Here's the drawing with two shaded views (mm, measured from the low corner). I have some questions. Give positions to 0.01 mm unless a question says otherwise; leave off trailing zeros. Write each loop counter-clockwise with the first axis right and the second up, starting at its lowest first coordinate (ties: lowest second). Pieces come first, ordered by that corner, then holes. Notation, with made-up numbers: (55.5, 54.5) - (90.5, 54.5) arc R38 cw to (90.5, 92.5) - close; hole circle Ø7 at (14, -31). An arc over 180 degrees is marked (long way). Answer as CSV lines item,"result". Start each with the question number.
Q1. Imagine slicing it at A-A on y = 17.5. List the corners of the cut face in (x, z) for me.
Q2. Will these pins go through, and if not, where does the flat tip stop? pin 1 Ø8 at (x, z) = (10, 7.5) entering from -Y; pin 2 Ø1.5 at (x, y) = (53, 35) entering from +Z (1 decimal); pin 3 Ø2 at (x, z) = (52, 21.5) entering from +Y; pin 4 Ø10 at (x, y) = (49.5, 12.5) entering from +Z (1 decimal).
Q3. Imagine slicing it at D-D on y = 7.5. List the corners of the cut face in (x, z) for me (1 decimal).
Q4. Imagine slicing it at C-C on x = 50. List the corners of the cut face in (y, z) for me.
Q5. If I drill on line 1 along Y through (x, z) = (29.5, 26); line 2 along X through (y, z) = (50.5, 18) (1 decimal); line 3 along X through (y, z) = (4, 4.5) (1 decimal), over which ranges is the centre line in solid material (lowest first)?
Q6. Imagine slicing it at B-B on z = 41. List the corners of the cut face in (x, y) for me (1 decimal).
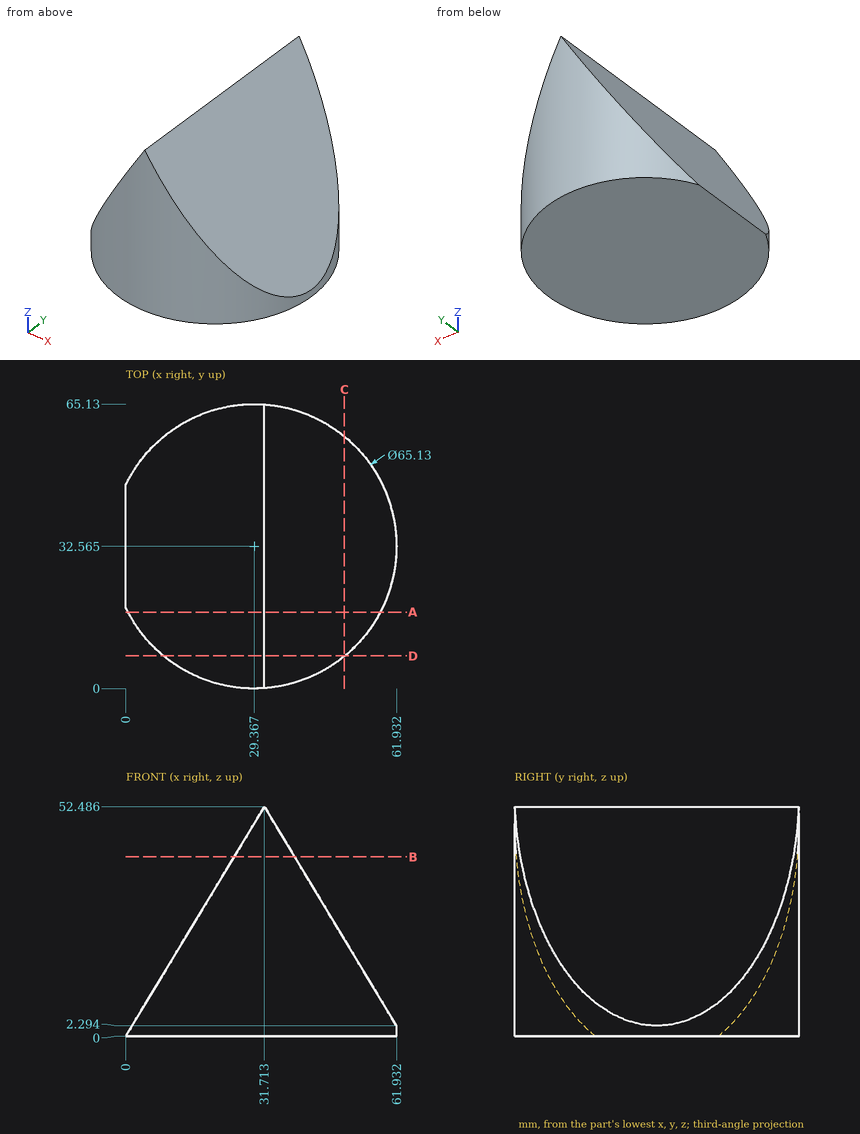
Conclusion:
1,outline,"(0.5, 0) - (58.24, 0) - (58.24, 8.43) - (31.71, 52.49) - (0.5, 0.82) - close"
2,pin 1,"y = 3.85"
2,pin 2,"z = 18.4"
2,pin 3,"through"
2,pin 4,"z = 31.2"
3,outline,"(8.6, 0) - (50.2, 0) - (50.2, 21.9) - (31.7, 52.5) - (8.6, 14.2) - close"
4,outline,"(7.37, 0) - (57.76, 0) - (57.76, 22.11) - (7.37, 22.11) - close"
5,line 1,"0 to 65.13"
5,line 2,"10.9 to 52.5"
5,line 3,"13.7 to 45"
6,outline,"(24.8, 0.3) arc R32.6 ccw to (38.6, 1.3) - (38.6, 63.8) arc R32.6 ccw to (24.8, 64.8) - close"
